from build123d import *

# Parameters (mm, degrees)
SKETCH_1_W                    = 60
SKETCH_1_H                    = 60
EXTRUDE_2_DEPTH               = 40
SKETCH_2_W                    = 40
SKETCH_2_H                    = 40
CUT_EXTRUDE_1_DEPTH           = 35
HOLE_WIZARD_12_0_12_1_D       = 12
HOLE_WIZARD_12_0_12_1_DEPTH   = 10
HOLE_WIZARD_13_5_13_5_1_D     = 13.5
HOLE_WIZARD_13_5_13_5_1_DEPTH = 10
HOLE_WIZARD_12_5_12_5_1_D     = 12.5
HOLE_WIZARD_12_5_12_5_1_DEPTH = 10
HOLE_WIZARD_13_0_13_1_D       = 13
HOLE_WIZARD_13_0_13_1_DEPTH   = 10


with BuildPart() as part:
    # 草圖1 → 填料-伸長2 (new body)
    with BuildSketch(Plane(origin=(0, 0, 0), x_dir=(1, 0, 0), z_dir=(0, 1, 0))):
        with Locations((-17.631578947, 47.236842105)):
            Rectangle(SKETCH_1_W, SKETCH_1_H)
    extrude(amount=EXTRUDE_2_DEPTH)

    # 草圖2 → 除料-伸長1 (cut)
    with BuildSketch(Plane(origin=(0, 40, 0), x_dir=(1, 0, 0), z_dir=(0, 1, 0))):
        with Locations((-17.631578947, 47.236842105)):
            Rectangle(SKETCH_2_W, SKETCH_2_H)
    extrude(amount=-CUT_EXTRUDE_1_DEPTH, mode=Mode.SUBTRACT)

    # Ø12.0 (12) 直徑孔1
    with Locations(Plane(origin=(-17.39385665, 23.867389925, -17.236842105), x_dir=(1, 0, 0), z_dir=(0, 0, 1))):
        with Locations((0, 0)):
            Hole(HOLE_WIZARD_12_0_12_1_D / 2, depth=HOLE_WIZARD_12_0_12_1_DEPTH)

    # Ø13.5 (13.5) 直徑孔1
    with Locations(Plane(origin=(12.368421053, 19.014409134, -48.421566687), x_dir=(0, 0, 1), z_dir=(1, 0, 0))):
        with Locations((0, 0)):
            Hole(HOLE_WIZARD_13_5_13_5_1_D / 2, depth=HOLE_WIZARD_13_5_13_5_1_DEPTH)

    # Ø12.5 (12.5) 直徑孔1
    with Locations(Plane(origin=(-47.631578947, 21.093271668, -46.835113177), x_dir=(0, 0, -1), z_dir=(-1, 0, 0))):
        with Locations((0, 0)):
            Hole(HOLE_WIZARD_12_5_12_5_1_D / 2, depth=HOLE_WIZARD_12_5_12_5_1_DEPTH)

    # Ø13.0 (13) 直徑孔1
    with Locations(Plane(origin=(-19.022665384, 20.011822427, -77.236842105), x_dir=(-1, 0, 0), z_dir=(0, 0, -1))):
        with Locations((0, 0)):
            Hole(HOLE_WIZARD_13_0_13_1_D / 2, depth=HOLE_WIZARD_13_0_13_1_DEPTH)


solid = part.part
Could you check a few things on this model? Use its own coordinates, in mm. A direction names the side the tool comes from. Give positions to 0.01 mm unless a question says otherwise; leave off trailing zeros. Order: outer loops, then holes, each group sorted by start corner. A loop starts at its lowest first (then second) coordinate and runs counter-clockwise, first axis right, second up. Notation, with made-up numbers: (81.5, 52.5) -> (92.5, 52.5) arc R5 ccw to (92.5, 59.5) -> close; hole circle Ø1 at (70, 86). An arc over 180 degrees is marked (long way). Return JSON: item names as keys, results as strings.
1. Imagine slicing it at C-C on z = -64. List the corners of the cut face in (x, y) for me.
Answer list:
{"outline": "(-47.63, 0) -> (12.37, 0) -> (12.37, 40) -> (2.37, 40) -> (2.37, 5) -> (-37.63, 5) -> (-37.63, 40) -> (-47.63, 40) -> close"}
2. Imagine slicing it at D-D on y = 22. List the corners of the cut face in (x, z) for me, then the cut area to 3 significant figures.
Answer list:
{"outline": "(-47.63, -77.24) -> (-25.21, -77.24) -> (-25.21, -67.24) -> (-37.63, -67.24) -> (-37.63, -53.02) -> (-47.63, -53.02) -> close; (-47.63, -40.65) -> (-37.63, -40.65) -> (-37.63, -27.24) -> (-23.1, -27.24) -> (-23.1, -17.24) -> (-47.63, -17.24) -> close; (-12.83, -77.24) -> (12.37, -77.24) -> (12.37, -54.48) -> (2.37, -54.48) -> (2.37, -67.24) -> (-12.83, -67.24) -> close; (-11.69, -27.24) -> (2.37, -27.24) -> (2.37, -42.37) -> (12.37, -42.37) -> (12.37, -17.24) -> (-11.69, -17.24) -> close", "area": "1,520 mm2"}
3. I need wall thicknesses on line 1 (X direction, y = 16.5, z = -61.5); line 2 (Z direction, x = 0, y = 17.5); line 3 (Y direction, x = -32, z = -32). Which ranges of each line are inside material? Lowest first, please. Write a range as from..to.
Answer list:
{"line 1": "x = -47.63..-37.63, 2.37..12.37", "line 2": "z = -77.24..-67.24, -27.24..-17.24", "line 3": "y = 0..5"}
4. Imagine slicing it at A-A on y = 7. List the corners of the cut face in (x, z) for me, then the cut area to 3 significant figures.
Answer list:
{"outline": "(-47.63, -77.24) -> (12.37, -77.24) -> (12.37, -17.24) -> (-47.63, -17.24) -> close; hole (-37.63, -67.24) -> (2.37, -67.24) -> (2.37, -27.24) -> (-37.63, -27.24) -> close", "area": "2,000 mm2"}
5. For pin 1 Ø11.5 at (x, y) = (-19.02, 20.01) entering from -Z, with a flat end and sliding along its axis, tell me the tip position at first contact or that it passes through.
Answer list:
{"pin 1": "stops at z = -27.24"}
6. On a 3-axis mill with a long thin cutter (end or side, diameter ignored), from which of +Z, -Z, +X, -X, +Y, -Y can I reach the whole of each face in a straight line? I mean faces 1 (the cylindrical face through (-42.562, 27.195, -48.19)), 2 (the cylindrical face through (-22.936, 21.569, -22.307)), 3 (the cylindrical face through (7.298, 18.718, -41.678)). Say none if no direction works.
Answer list:
{"face 1": "-X", "face 2": "+Z", "face 3": "+X"}
7. Thinking about a two-plate mould opening in Y: for faces 4 (the flat face through (-38, 40, -48)), 5 (the cylindrical face through (-23.813, 24.405, -72.167)), 6 (the flat face through (2.368, 27, -47)), 7 (the flat face through (-18, 0, -48)), which applies, pulls with the +Y half, pulls with the -Y half, needs draft (parallel to the pull), parting line crosses it, or undercut?
Answer list:
{"face 4": "pulls with the +Y half", "face 5": "undercut", "face 6": "needs draft", "face 7": "pulls with the -Y half"}
8. Imagine slicing it at B-B on x = -8. List the corners of the cut face in (y, z) for me.
Answer list:
{"outline": "(0, -77.24) -> (40, -77.24) -> (40, -67.24) -> (5, -67.24) -> (5, -27.24) -> (40, -27.24) -> (40, -17.24) -> (0, -17.24) -> close"}
